For this review, use the dimensioned drawing (mm, ordinates from the lowest corner) and the shaded views. Give positions to 0.01 mm unless a question says otherwise; leave off trailing zeros. Loops run counter-clockwise (first coordinate to the right, second up) from the corner with the lowest first, then second, coordinate; pieces in that order, holes last. Notation, with made-up numbers: M 10.5,-37 L 54.5,-37 A26 ccw 54.5,-21 Z; hole C 7.5,-35.75 d6. An arc over 180 degrees is marked long. Use CSV: the item, a comma, the result in double quotes.
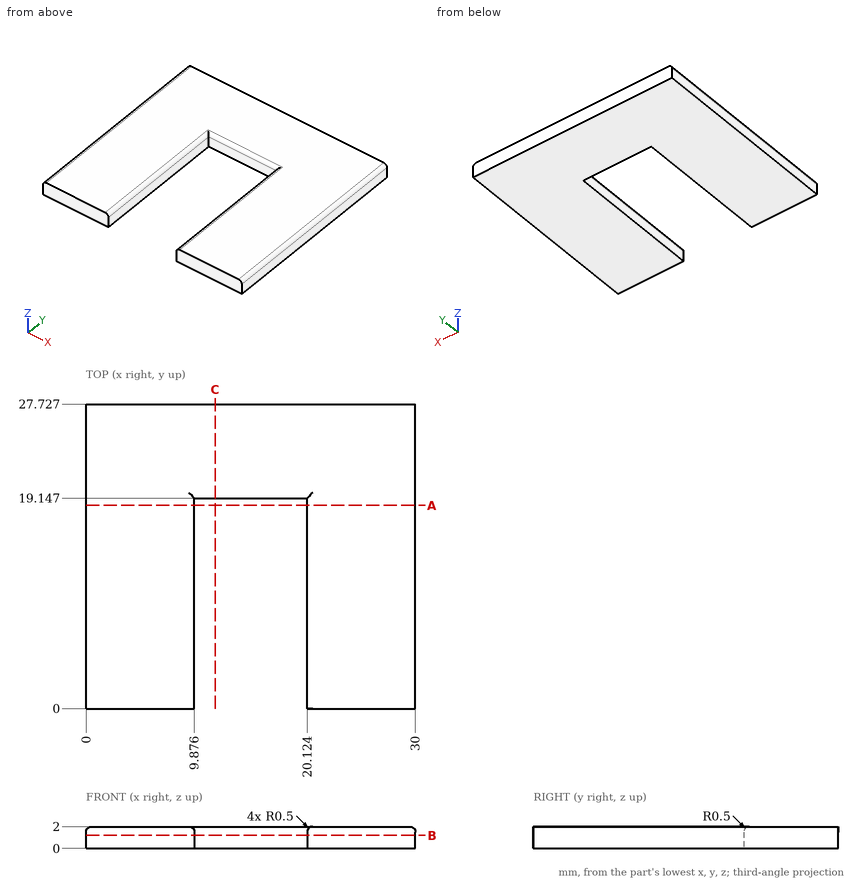
(1) We need section C-C on x = 11.75. State the section outline as (y, z) points, then the cut area to 3 significant figures.
A:
outline,"M 19.15,0 L 27.73,0 L 27.73,2 L 19.65,2 A0.5 ccw 19.15,1.5 Z"
area,"17.1 mm²"
(2) Wall thickness on line 1 along X through (y, z) = (9, 1.55); line 2 along X through (y, z) = (17, 1.9) (1 decimal); line 3 along Y through (x, z) = (11.75, 1.6): over which ranges is each line inside the solid? List them lowest first. Write a range as [from, to].
A:
line 1,"[0, 9.87], [20.13, 30]"
line 2,"[0.2, 9.7], [20.3, 29.8]"
line 3,"[19.16, 27.73]"
(3) We need section B-B on z = 1.2. State the section outline as (x, y) points (1 decimal).
A:
outline,"M 0,0 L 9.9,0 L 9.9,19.1 L 20.1,19.1 L 20.1,0 L 30,0 L 30,27.7 L 0,27.7 Z"
(4) Clearance check with a flat-ended pin moving along its axis: P1, Ø0.8, axis at x = 15.5, z = 1, coming from the -Y side. State where the tip first meets the part, or that it passes through.
A:
P1,"y = 19.15"
(5) We need section A-A on y = 18.5. State the section outline as (x, z) points (1 decimal).
A:
outline,"M 0,0 L 9.9,0 L 9.9,1.5 A0.5 ccw 9.4,2 L 0.5,2 A0.5 ccw 0,1.5 Z; M 20.1,0 L 30,0 L 30,1.5 A0.5 ccw 29.5,2 L 20.6,2 A0.5 ccw 20.1,1.5 Z"
